CAD build for the part. Positions are in the model's coordinates, mm. Coordinates: 2 decimals unless noted, no trailing zeros. Order: outer loops, then holes, each group sorted by start corner. A loop starts at its lowest first (then second) coordinate and runs counter-clockwise, first axis right, second up. Notation, with made-up numbers: M -28,29.25 L 6,29.25 A15 ccw 6,39.25 Z; hole C 21.5,-33 d2. An arc over 180 degrees is marked long. One line per item, written item: value.
from build123d import *

# Parameters (mm, degrees)
SKETCH2_W           = 3.175
SKETCH2_H           = 28.055216984
BOSS_EXTRUDE1_DEPTH = 5.08
CHAMFER1_SIZE       = 5.08


with BuildPart() as part:
    # Sketch2 → Boss-Extrude1 (new body)
    with BuildSketch(Plane(origin=(0, 1065.810275743, -19.39007848), x_dir=(1, 0, 0), z_dir=(4.449407192603594e-15, 0.9998345519923184, -0.018189795004890538))):
        with Locations((671.194724889, -1291.239942416)):
            Rectangle(SKETCH2_W, SKETCH2_H)
    extrude(amount=BOSS_EXTRUDE1_DEPTH)

    # Chamfer1
    chamfer1_edges = [part.edges().sort_by_distance(p)[0] for p in [
        (671.194724889, 1094.631984445, 1285.569114354),
    ]]
    chamfer(chamfer1_edges, length=CHAMFER1_SIZE - 0.0001)  # a hair under: the kernel refuses the full size


solid = part.part
Q1. Drill centre lines: line 1 along Y through (x, z) = (672.1, 1280.25); line 2 along Y through (x, z) = (670.15, 1269.75); line 3 along Z through (x, y) = (670.1, 1093.35). Where is each one in solid material? Low to high.
Recorded:
line 1: y = 1089.45 to 1094.54
line 2: y = 1089.26 to 1094.34
line 3: z = 1257.53 to 1281.72
Q2. Slice it at B-B (z = 1283.75). List the corners of the cut face in (x, y), plus the area to 3 significant figures.
Recorded:
outline: M 669.61,1089.52 L 672.78,1089.52 L 672.78,1091.4 L 669.61,1091.4 Z
area: 5.96 mm^2
Q3. Slice it at C-C (y = 1092.2). List the corners of the cut face in (x, z), plus the area to 3 significant figures.
Recorded:
outline: M 669.61,1257.55 L 672.78,1257.55 L 672.78,1282.92 L 669.61,1282.92 Z
area: 80.5 mm^2
